```python
from build123d import *

# Parameters (mm, degrees)
F0_W     = 90
F0_H     = 50
F0_R     = 5.9031202678
F0_R_2   = 6.221473217
F2_DEPTH = 10
F1_W     = 26.3143666089
F1_H     = 50
F3_DEPTH = 15
F4_R     = 5
F5_D     = 14
F5_DEPTH = 5
F5_TIP   = 4.2060243332
F6_D     = 5


with BuildPart() as f2:
    # F0 (on Top) → F2 (new body)
    with BuildSketch(Plane.XY):
        with Locations((1.7176882843, 25)):
            Rectangle(F0_W, F0_H)
        with Locations((-30.9307053685, 40.3467603028)):
            Circle(F0_R, mode=Mode.SUBTRACT)
        with Locations((34.2310518026, 41.3290970027)):
            Circle(F0_R_2, mode=Mode.SUBTRACT)
    extrude(amount=-F2_DEPTH)

    # F1 (on Front) → F3 (join)
    with BuildSketch(Plane.XZ):
        with Locations((0, 25)):
            Rectangle(F1_W, F1_H)
        with BuildLine():
            Line((-13.1571833044, 50), (13.1571833044, 50))
            ThreePointArc((13.1571833044, 50), (0, 63.1571833044), (-13.1571833044, 50))
        make_face()
    extrude(amount=-F3_DEPTH)

    # F4
    f4_edges = [f2.edges().sort_by_distance(p)[0] for p in [
        (46.717688, 0, -5),
        (46.717688, 50, -5),
        (-43.282312, 50, -5),
        (-43.282312, 0, -5),
    ]]
    fillet(f4_edges, radius=F4_R)

    # F5
    with Locations(Plane.XZ):
        with Locations((0, 50)):
            Hole(F5_D / 2, depth=F5_DEPTH)
            with Locations((0, 0, -(F5_DEPTH + F5_TIP / 2))):  # 118° drill point
                Cone(0, F5_D / 2, F5_TIP, mode=Mode.SUBTRACT)

    # F6 (through all)
    with Locations(Plane.XZ):
        with Locations((0, 50)):
            Hole(F6_D / 2)


solid = f2.part
```
Input: part model. Units: mm. Frame: model coordinates. A direction names the side the tool comes from. Coordinates: 2 decimals unless noted, no trailing zeros. Loops run counter-clockwise (first coordinate to the right, second up) from the corner with the lowest first, then second, coordinate; pieces in that order, holes last. Notation, with made-up numbers: (68, 39) -> (116, 39) arc R10 cw to (116, 52) -> close; hole circle Ø8 at (76, 88.25). An arc over 180 degrees is marked (long way). Use a Markdown table: item, result.
1) Pull-direction query (Z, two-part tool) for faces 4 (the flat face through (1, 0, 19)), 5 (the cylindrical face through (0.91, 2.54, 56.94)), 6 (the flat face through (1, 25, -10)); classes: released by +Z, released by -Z, zero draft, split by the parting line, or undercut.
Results found:
| item | result |
|---|---|
| face 4 | zero draft |
| face 5 | undercut |
| face 6 | released by -Z |
2) Cut plane A-A (x = 0). Return the cut outline in (y, z).
Results found:
| item | result |
|---|---|
| outline | (0, -10) -> (50, -10) -> (50, 0) -> (15, 0) -> (15, 47.5) -> (7.7, 47.5) -> (5, 43) -> (0, 43) -> close; (0, 57) -> (5, 57) -> (7.7, 52.5) -> (15, 52.5) -> (15, 63.16) -> (0, 63.16) -> close |
3) Contact query for flat-ended pins moving along their axis: pin 1 (5 mm diameter, centred on x = -23, z = 3, fed in from +Y); pin 2 (6.5 mm diameter, centred on x = 0, z = 50, fed in from +Y); pin 3 (11 mm diameter, centred on x = 0, z = 50, fed in from -Y); pin 4 (2 mm diameter, centred on x = -8, y = 13, fed in from +Z). Output: stop coordinate, or through.
Results found:
| item | result |
|---|---|
| pin 1 | passes through |
| pin 2 | stops at y = 15 |
| pin 3 | stops at y = 5.9 |
| pin 4 | stops at z = 61.14 |
4) Material intervals for line 1 along Z through (x, y) = (0, 11.75); line 2 along X through (y, z) = (13, 50); line 3 along X through (y, z) = (5.5, 16), sorted ascending. Write a range as from..to.
Results found:
| item | result |
|---|---|
| line 1 | z = -10..47.5, 52.5..63.16 |
| line 2 | x = -13.16..-2.5, 2.5..13.16 |
| line 3 | x = -13.16..13.16 |
5) Access query for faces 1 (the flat face through (0, 15, 32)), 2 (the flat face through (-13.157, 7, 25)), 3 (the flat face through (13.157, 7, 25)). Directions: +Z, -Z, +X, -X, +Y, -Y. A direction counts if a zero-diameter tool reaches every point of the face in a straight line with its end or side. Return the directions, or none.
Results found:
| item | result |
|---|---|
| face 1 | +Z, +X, -X, +Y |
| face 2 | +Z, -X, +Y, -Y |
| face 3 | +Z, +X, +Y, -Y |
6) Cut plane D-D (y = 18.5). Return the cut outline in (x, z), then the cut area to 3 significant figures.
Results found:
| item | result |
|---|---|
| outline | (-43.28, -10) -> (46.72, -10) -> (46.72, 0) -> (-43.28, 0) -> close |
| area | 900 mm2 |
7) Cut plane B-B (z = 40.5). Return the cut outline in (x, y), then the cut area to 3 significant figures.
Results found:
| item | result |
|---|---|
| outline | (-13.16, 0) -> (13.16, 0) -> (13.16, 15) -> (-13.16, 15) -> close |
| area | 395 mm2 |
8) Cut plane C-C (x = -29.5). Return the cut outline in (y, z).
Results found:
| item | result |
|---|---|
| outline | (0, -10) -> (34.62, -10) -> (34.62, 0) -> (0, 0) -> close; (46.07, -10) -> (50, -10) -> (50, 0) -> (46.07, 0) -> close |
